Read the model definition and answer for the solid it produces. Units are mm, in the model's axes. Face numbers are marked on the shaded views. Coordinates: 2 decimals unless noted, no trailing zeros. Answer as a JSON object with one key per item and string values. Group by question number.
Q1. Straight lines are drawn through the part: line 1 along Y through (x, z) = (0, 0.5) (3 decimals); line 2 along Y through (x, z) = (-29.5, 4); line 3 along Y through (x, z) = (3, 0). For each, find the intervals that lie inside material, in ascending order. Write a range as [from, to].
Q2. The part is cut by section A-A on z = 3.5. State how many separate pieces and enclosed holes the cut face has, and give its area (3 significant figures).
Q3. Each of these flat-tipped pins is pushed along its axis until it touches: P1, Ø8, axis at x = -94, z = 3.5, coming from the +Y side; P2, Ø4, axis at x = 30.5, z = 4, coming from the -Y side; P3, Ø12.5, axis at x = 91, z = 1.5, coming from the +Y side; P4, Ø2, axis at x = 0, y = -7, coming from the -Z side (3 decimals). Where does it stop, or does it pass through?
Q4. Determine the mould class of the marked faces 1 and 2 for opening direction X: released by +X, released by -X, zero draft, split by the parting line, or undercut.
from build123d import *

# Parameters (mm, degrees)
BOSS_EXTRUDE1_DEPTH      = 50
BOSS_EXTRUDE1_DEPTH_BACK = 5
SKETCH2_R                = 215
SKETCH2_R_2              = 205
BOSS_EXTRUDE2_DEPTH      = 20
BOSS_EXTRUDE2_DEPTH_BACK = 5
SKETCH3_R                = 1
FILLET1_R                = 5
FILLET2_R                = 5
SCALE1_SCALE             = 0.625


with BuildPart() as part:
    # Sketch2 → Boss-Extrude1 (new, two sides: drawn at the far end of the back side and taken through both)
    with BuildSketch(Plane.XY.offset(-BOSS_EXTRUDE1_DEPTH_BACK)):
        Circle(SKETCH2_R)
        Circle(SKETCH2_R_2, mode=Mode.SUBTRACT)
    extrude(amount=BOSS_EXTRUDE1_DEPTH + BOSS_EXTRUDE1_DEPTH_BACK)

    # Sketch3 → Boss-Extrude2 (add, two sides: drawn at the far end of the back side and taken through both)
    with BuildSketch(Plane.XY.offset(-BOSS_EXTRUDE2_DEPTH_BACK)):
        with BuildLine():
            Line((210.976119612, 2.604722665), (14.772116295, 2.604722665))
            ThreePointArc((14.772116295, 2.604722665), (10.606601718, 10.606601718), (2.604722665, 14.772116295))
            Line((2.604722665, 14.772116295), (2.604722665, 210.976119612))
            Line((2.604722665, 210.976119612), (-2.604722665, 210.976119612))
            Line((-2.604722665, 210.976119612), (-2.604722665, 14.772116295))
            ThreePointArc((-2.604722665, 14.772116295), (-10.606601718, 10.606601718), (-14.772116295, 2.604722665))
            Line((-14.772116295, 2.604722665), (-210.976119612, 2.604722665))
            Line((-210.976119612, 2.604722665), (-210.976119612, -2.604722665))
            Line((-210.976119612, -2.604722665), (-14.772116295, -2.604722665))
            ThreePointArc((-14.772116295, -2.604722665), (-10.606601718, -10.606601718), (-2.604722665, -14.772116295))
            Line((-2.604722665, -14.772116295), (-2.604722665, -210.976119612))
            Line((-2.604722665, -210.976119612), (2.604722665, -210.976119612))
            Line((2.604722665, -210.976119612), (2.604722665, -14.772116295))
            ThreePointArc((2.604722665, -14.772116295), (10.606601718, -10.606601718), (14.772116295, -2.604722665))
            Line((14.772116295, -2.604722665), (210.976119612, -2.604722665))
            Line((210.976119612, -2.604722665), (210.976119612, 2.604722665))
        make_face()
        with Locations((0, -11.2)):
            Circle(SKETCH3_R, mode=Mode.SUBTRACT)
        with Locations((-11.2, 0)):
            Circle(SKETCH3_R, mode=Mode.SUBTRACT)
        with BuildLine():
            ThreePointArc((-5.514923417, -0.972429795), (-5.6, 0), (-5.514923417, 0.972429795))
            ThreePointArc((-5.514923417, 0.972429795), (-3.959797975, 3.959797975), (-0.972429795, 5.514923417))
            ThreePointArc((-0.972429795, 5.514923417), (0, 5.6), (0.972429795, 5.514923417))
            ThreePointArc((0.972429795, 5.514923417), (3.959797975, 3.959797975), (5.514923417, 0.972429795))
            ThreePointArc((5.514923417, 0.972429795), (5.578690309, 0.488072159), (5.6, 0))
            ThreePointArc((5.6, 0), (5.578690309, -0.488072159), (5.514923417, -0.972429795))
            ThreePointArc((5.514923417, -0.972429795), (3.959797975, -3.959797975), (0.972429795, -5.514923417))
            ThreePointArc((0.972429795, -5.514923417), (0, -5.6), (-0.972429795, -5.514923417))
            ThreePointArc((-0.972429795, -5.514923417), (-3.959797975, -3.959797975), (-5.514923417, -0.972429795))
        make_face(mode=Mode.SUBTRACT)
        with Locations((11.2, 0)):
            Circle(SKETCH3_R, mode=Mode.SUBTRACT)
        with Locations((0, 11.2)):
            Circle(SKETCH3_R, mode=Mode.SUBTRACT)
    extrude(amount=BOSS_EXTRUDE2_DEPTH + BOSS_EXTRUDE2_DEPTH_BACK)

    # Fillet1
    fillet1_edges = [part.edges().sort_by_distance(p)[0] for p in [
        (-215, 0, 50),
    ]]
    fillet(fillet1_edges, radius=FILLET1_R)

    # Fillet2
    # the kernel refuses this fillet: 5 mm, written as the material it takes off along each edge
    with BuildSketch(Plane(origin=(0, 0, -5), x_dir=(1, 0, 0), z_dir=(0, -1, 0))) as fillet2_piece_1:
        with BuildLine():
            CenterArc((215 - FILLET2_R, FILLET2_R), FILLET2_R, 270, 90)
            Line((215 - FILLET2_R, 0), (215, 0))
            Line((215, 0), (215, FILLET2_R))
        make_face()
    revolve(axis=Axis((0, 0, -5), (0, 0, 1)), mode=Mode.SUBTRACT)


with BuildPart() as part_1:
    # Scale1: scaled about (0, 0, 0)
    add(part.part.scale(SCALE1_SCALE))


solid = part_1.part
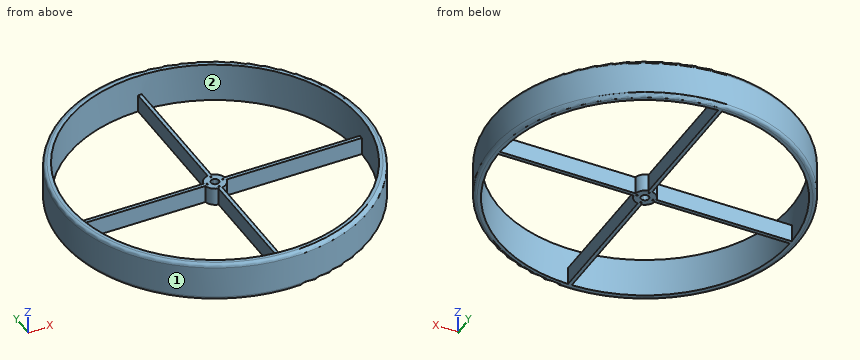
Final values:
{
 "1": {"line 1": "y = [-134.375, -7.625], [-6.375, -3.5], [3.5, 6.375], [7.625, 134.375]", "line 2": "y = [-131.1, -124.68], [-1.63, 1.63], [124.68, 131.1]", "line 3": "y = [-134.34, -128.09], [-8.88, -1.8], [1.8, 8.88], [128.09, 134.34]"},
 "2": {"separate pieces": "1", "enclosed holes": "9", "area": "6,930 mm2"},
 "3": {"P1": "stops at y = 99.78", "P2": "stops at y = -131.32", "P3": "stops at y = 104.28", "P4": "stops at z = -3.125"},
 "4": {"face 1": "split by the parting line", "face 2": "undercut"}
}
